from build123d import *

# Parameters (mm, degrees)
SKETCH1_R                   = 12
EXTRUDE1_DEPTH              = 180
M6_TAPPED_HOLE1_D           = 5
M6_TAPPED_HOLE1_DEPTH       = 15
M6_TAPPED_HOLE1_CBORE_D     = 6
M6_TAPPED_HOLE1_CBORE_DEPTH = 12
M6_TAPPED_HOLE1_TIP         = 1.502151548


with BuildPart() as part:
    # Sketch1 → Extrude1 (new body)
    with BuildSketch(Plane(origin=(0, 0, 0), x_dir=(1, 0, 0), z_dir=(0, 1, 0))):
        with Locations(Location((0, 0, 0), (0, 0, 270))):
            Circle(SKETCH1_R)
    extrude(amount=-EXTRUDE1_DEPTH)

    # M6 Tapped Hole1
    with Locations(Plane(origin=(0, 0, 0), x_dir=(-1, 0, 0), z_dir=(0, 1, 0))):
        with Locations((0, 0)):
            CounterBoreHole(M6_TAPPED_HOLE1_D / 2, M6_TAPPED_HOLE1_CBORE_D / 2, M6_TAPPED_HOLE1_CBORE_DEPTH, depth=M6_TAPPED_HOLE1_DEPTH)
            with Locations((0, 0, -(M6_TAPPED_HOLE1_DEPTH + M6_TAPPED_HOLE1_TIP / 2))):  # 118° drill point
                Cone(0, M6_TAPPED_HOLE1_D / 2, M6_TAPPED_HOLE1_TIP, mode=Mode.SUBTRACT)


solid = part.part
The listing builds one solid part. Answer for the finished solid, in the listing's coordinates (mm). A direction names the side the tool comes from. Coordinates: 2 decimals unless noted, no trailing zeros. Loops run counter-clockwise (first coordinate to the right, second up) from the corner with the lowest first, then second, coordinate; pieces in that order, holes last. Notation, with made-up numbers: (56, 70.25) -> (115, 70.25) arc R28 cw to (115, 96.25) -> close; hole circle Ø4 at (-18.75, 38). An arc over 180 degrees is marked (long way). Answer in a Markdown table with one row per item. Add a question column.
1. Determine the mould class of faces 3 (the flat face through (2, -12, 2)), 4 (the flat face through (0, -180, 0)), 5 (the conical face through (0.094, -16.241, -0.424)), 6 (the cylindrical face through (3.604, -88.74, 11.446)) for opening direction X: +X half, -X half, draft (parallel to the pull), parting line (faces both ways), or undercut.
2. Consider line 1 (X direction, y = -13, z = 0); line 2 (X direction, y = -48, z = 0.25); line 3 (Z direction, x = 10.25, y = -104.5). Determine where each line is inside the solid, lowest interval first. Write a range as [from, to].
3. The part is cut by section B-B, the plane x = -9.75. Write down the section's boundary in (y, z), then the cut area to 3 significant figures.
4. For faces 1 (the flat face through (-2.5, 0, 2.5)), 2 (the cylindrical face through (3, -6, 0)), determine the directions among +Z, -Z, +X, -X, +Y, -Y from which every point of the face is accessible in a straight line to the end or side of a thin tool.
5. The part is cut by section A-A, the plane y = -137. Write down the section's boundary in (x, z), then the cut area to 3 significant figures.
6. Flat-ended cylindrical pins translate along their axes: P1, Ø5.5, axis at x = 0, z = 0, coming from the +Y side; P2, Ø5, axis at x = -9, y = -94.5, coming from the +Z side; P3, Ø1.8, axis at x = -1.5, z = 0, coming from the +Y side. Find the tip coordinate at first contact, or state that the pin passes through.
7. The part is cut by section C-C, the plane z = -8.75. Write down the section's boundary in (x, y).
Answer below:
| question | item | result |
|---|---|---|
| 1 | face 3 | undercut |
| 1 | face 4 | draft |
| 1 | face 5 | undercut |
| 1 | face 6 | parting line |
| 2 | line 1 | [-12, -2.5], [2.5, 12] |
| 2 | line 2 | [-12, 12] |
| 2 | line 3 | [-6.24, 6.24] |
| 3 | outline | (-180, -7) -> (0, -7) -> (0, 7) -> (-180, 7) -> close |
| 3 | area | 2,520 mm2 |
| 4 | face 1 | +Z, -Z, +X, -X, +Y |
| 4 | face 2 | +Y |
| 5 | outline | circle Ø24 at (0, 0) |
| 5 | area | 452 mm2 |
| 6 | P1 | y = -12 |
| 6 | P2 | z = 10.09 |
| 6 | P3 | y = -15.06 |
| 7 | outline | (-8.21, -180) -> (8.21, -180) -> (8.21, 0) -> (-8.21, 0) -> close |
